The listing builds one solid part. Answer for the finished solid, in the listing's coordinates (mm). Face numbers are marked on the shaded views. A direction names the side the tool comes from. Give positions to 0.01 mm unless a question says otherwise; leave off trailing zeros. Write each loop counter-clockwise with the first axis right and the second up, starting at its lowest first coordinate (ties: lowest second). Pieces come first, ordered by that corner, then holes. Notation, with made-up numbers: M 75.25,44 L 95.25,44 A26 cw 95.25,78 Z; hole C -37.75,23 d5. An arc over 180 degrees is marked long. Return JSON: item names as keys, results as strings.
from build123d import *

# Parameters (mm, degrees)
SKETCH1_R                = 19
SKETCH1_R_2              = 7.5
SKETCH1_R_3              = 2.5
BOSS_EXTRUDE5_DEPTH      = 2
SKETCH10_R               = 12
CUT_EXTRUDE33_DEPTH      = 1
CUT_EXTRUDE34_DEPTH      = 40
CUT_EXTRUDE34_DEPTH_BACK = 34
SKETCH14_R               = 0.6


with BuildPart() as part:
    # Sketch1 → Boss-Extrude5 (new body)
    # profile 1 of 2: a face of its own
    with BuildSketch(Plane.XY):
        Circle(SKETCH1_R)
        Circle(SKETCH1_R_2, mode=Mode.SUBTRACT)
    # profile 2 of 2: a face of its own
    with BuildSketch(Plane.XY):
        Circle(SKETCH1_R_2)
        Circle(SKETCH1_R_3, mode=Mode.SUBTRACT)
    extrude(amount=BOSS_EXTRUDE5_DEPTH)

    # Sketch10 → Cut-Extrude33 (cut)
    with BuildSketch(Plane.XY):
        Circle(SKETCH10_R)
    extrude(amount=CUT_EXTRUDE33_DEPTH, mode=Mode.SUBTRACT)

    # Sketch14 → Cut-Extrude34 (cut, two sides: drawn at the far end of the back side and taken through both)
    with BuildSketch(Plane(origin=(0, 0, 0), x_dir=(0, 0, -1), z_dir=(1, 0, 0)).offset(-CUT_EXTRUDE34_DEPTH_BACK)):
        with Locations(Location((-1.062968904, 4, 0), (0, 0, 180))):
            Circle(SKETCH14_R)
        with Locations(Location((-1.062968904, -4, 0), (0, 0, 180))):
            Circle(SKETCH14_R)
    extrude(amount=CUT_EXTRUDE34_DEPTH + CUT_EXTRUDE34_DEPTH_BACK, mode=Mode.SUBTRACT)


solid = part.part
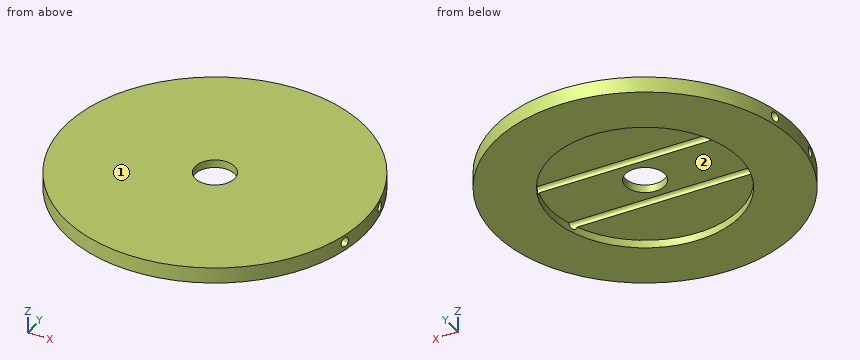
Item 1: Which of the six approach directions +Z, -Z, +X, -X, +Y, -Y give full straight-line access (tool end or side, diameter ignored) to the marked faces 1 and 2?
Geometry results:
{"face 1": "+Z, +X, -X, +Y, -Y", "face 2": "-Z"}
Item 2: A cutting plane is placed at C-C, the plane y = -2. Write down the section's boundary in (x, z), plus the area to 3 significant figures.
Geometry results:
{"outline": "M -18.89,0 L -11.83,0 L -11.83,1 L -1.5,1 L -1.5,2 L -18.89,2 Z; M 1.5,1 L 11.83,1 L 11.83,0 L 18.89,0 L 18.89,2 L 1.5,2 Z", "area": "48.9 mm2"}
Item 3: Given pin 1 Ø2 at (x, y) = (-3.5, 0) entering from -Z; pin 2 Ø1 at (y, z) = (4, 1.06) entering from -X, each flat-ended and moving along its own axis, determine where each tip first touches the part or whether it passes through.
Geometry results:
{"pin 1": "stops at z = 1", "pin 2": "passes through"}
Item 4: A cutting plane is placed at B-B, the plane y = 4. Write down the section's boundary in (x, z).
Geometry results:
{"outline": "M -18.57,0 L -11.31,0 L -11.31,0.46 L -18.57,0.46 Z; M -18.57,1.66 L 18.57,1.66 L 18.57,2 L -18.57,2 Z; M 11.31,0 L 18.57,0 L 18.57,0.46 L 11.31,0.46 Z"}
Item 5: A cutting plane is placed at A-A, the plane x = 0. Write down the section's boundary in (y, z).
Geometry results:
{"outline": "M -19,0 L -12,0 L -12,1 L -4.6,1 A0.6 cw long -3.4,1 L -2.5,1 L -2.5,2 L -19,2 Z; M 2.5,1 L 3.4,1 A0.6 cw long 4.6,1 L 12,1 L 12,0 L 19,0 L 19,2 L 2.5,2 Z"}
Item 6: Find the intervals of material crossed by line 1 (Y direction, x = 0, z = 1.75); line 2 (Y direction, x = -3, z = 1.3); line 3 (Y direction, x = 12.5, z = 1.1), in increasing order.
Geometry results:
{"line 1": "y = -19 to -2.5, 2.5 to 19", "line 2": "y = -18.76 to -4.55, -3.45 to 3.45, 4.55 to 18.76", "line 3": "y = -14.31 to -4.6, -3.4 to 3.4, 4.6 to 14.31"}
Item 7: A cutting plane is placed at D-D, the plane x = -10.5. Write down the section's boundary in (y, z), plus the area to 3 significant figures.
Geometry results:
{"outline": "M -15.84,0 L -5.81,0 L -5.81,1 L -4.6,1 A0.6 cw long -3.4,1 L 3.4,1 A0.6 cw long 4.6,1 L 5.81,1 L 5.81,0 L 15.84,0 L 15.84,2 L -15.84,2 Z", "area": "50.4 mm2"}
